Model file for the job. Use its own axes, mm. A direction names the side the tool comes from. Round coordinates to 2 decimals unless told otherwise and drop trailing zeros. Loops run counter-clockwise (first coordinate to the right, second up) from the corner with the lowest first, then second, coordinate; pieces in that order, holes last. Notation, with made-up numbers: (79.25, -4.75) - (107.25, -4.75) arc R17 cw to (107.25, 16.25) - close; hole circle Ø3 at (22, 26). An arc over 180 degrees is marked (long way). Answer as a JSON object with one key per item and string values.
Autodesk Inventor part; units mm, degrees
ref_plane "YZ Plane" through (0, 0, 0) normal (1, 0, 0) x (0, 1, 0)
ref_plane "XZ Plane" through (0, 0, 0) normal (0, 1, 0) x (-1, 0, 0)
ref_plane "XY Plane" through (0, 0, 0) normal (0, 0, 1) x (1, 0, 0)
sketch "Esquisse1" plane through (0, 0, 0) normal (0, 0, 1) x (1, 0, 0)
  line L0 (33.2, -53.2) -> (-33.2, -53.2)
  line L1 (-33.2, -53.2) -> (-33.2, 53.2)
  line L2 (-33.2, 53.2) -> (33.2, 53.2)
  line L3 (33.2, 53.2) -> (33.2, -53.2)
  line L4 (33.2, -53.2) -> (-33.2, 53.2) construction
  line L5 (-33.2, -53.2) -> (33.2, 53.2) construction
  line L6 (30.2, 50.2) -> (-30.2, 50.2)
  line L7 (-30.2, 50.2) -> (-30.2, -50.2)
  line L8 (-30.2, -50.2) -> (30.2, -50.2)
  line L9 (30.2, -50.2) -> (30.2, 50.2)
  point P0 (0, 0)
  dimension "d0" = 66.4
  dimension "d1" = 106.4
  dimension "d2" = 3
extrude "Extrusion1" add sketch "Esquisse1" along normal blind 1.6
fillet "Congé1" radius 11 4 edges at (-33.2, 53.2, 0.8) (33.2, 53.2, 0.8) (33.2, -53.2, 0.8) (-33.2, -53.2, 0.8)
fillet "Congé1" radius 8 4 edges at (30.2, -50.2, 0.8) (-30.2, -50.2, 0.8) (-30.2, 50.2, 0.8) (30.2, 50.2, 0.8)
chamfer "Chanfrein1" distance 2.2 distance2 1.15 8 edges at (-33.2, 0, 1.6) (-29.9782, -49.9782, 1.6) (0, -53.2, 1.6) (29.9782, -49.9782, 1.6) (33.2, 0, 1.6) (29.9782, 49.9782, 1.6) (0, 53.2, 1.6) (-29.9782, 49.9782, 1.6) measured on face at (-31.2, 14.0667, 1.6)
properties part number "FrontPanelBezel"
1) Drop a flat-ended pin along its axis: P1, Ø0.5, axis at x = 9, z = 1, coming from the -Y side. Give the stop position or say it passes through.
Values follow:
{"P1": "y = -52.63"}
2) Probe probe 1 along Y at (x, z) = (11, 0.4); probe 2 along X at (y, z) = (-21, 0.35); probe 3 along Y at (x, z) = (-2.5, 0.5). List the from-to ranges inside material, lowest first.
Values follow:
{"probe 1": "-53.2 to -50.2, 50.2 to 53.2", "probe 2": "-33.2 to -30.2, 30.2 to 33.2", "probe 3": "-53.1 to -50.2, 50.2 to 53.1"}
3) Slice it at C-C on z = 1.1. List the corners of the cut face in (x, y).
Values follow:
{"outline": "(-31.96, -42.2) arc R9.76 ccw to (-22.2, -51.96) - (22.2, -51.96) arc R9.76 ccw to (31.96, -42.2) - (31.96, 42.2) arc R9.76 ccw to (22.2, 51.96) - (-22.2, 51.96) arc R9.76 ccw to (-31.96, 42.2) - close; hole (-30.2, -42.2) arc R8 ccw to (-22.2, -50.2) - (22.2, -50.2) arc R8 ccw to (30.2, -42.2) - (30.2, 42.2) arc R8 ccw to (22.2, 50.2) - (-22.2, 50.2) arc R8 ccw to (-30.2, 42.2) - close"}
4) Slice it at A-A on y = -33. List the corners of the cut face in (x, z), then the cut area to 3 significant figures.
Values follow:
{"outline": "(-33.2, 0) - (-30.2, 0) - (-30.2, 1.6) - (-31, 1.6) - (-33.2, 0.45) - close; (30.2, 0) - (33.2, 0) - (33.2, 0.45) - (31, 1.6) - (30.2, 1.6) - close", "area": "7.07 mm²"}
5) Slice it at B-B on x = -18.5. List the corners of the cut face in (y, z).
Values follow:
{"outline": "(-53.2, 0) - (-50.2, 0) - (-50.2, 1.6) - (-51, 1.6) - (-53.2, 0.45) - close; (50.2, 0) - (53.2, 0) - (53.2, 0.45) - (51, 1.6) - (50.2, 1.6) - close"}
6) Tool access for faces 1 (the conical face through (28.62, 48.76, 1.4)), 2 (the cylindrical face through (-27.919, -47.794, 0.811)): list every direction of +Z, -Z, +X, -X, +Y, -Y with a clear straight run to the whole face (end or side of a thin tool).
Values follow:
{"face 1": "+Z, +X, +Y", "face 2": "+Z, -Z"}
